Source: CAD feature listing. Evaluate the final solid. Frame: model axes, mm. Face numbers are marked on the shaded views. A direction names the side the tool comes from. Give positions to 0.01 mm unless a question says otherwise; leave off trailing zeros. Write each loop counter-clockwise with the first axis right and the second up, starting at its lowest first coordinate (ties: lowest second). Pieces come first, ordered by that corner, then holes.
```python
from build123d import *

# Parameters (mm, degrees)
SKETCH1_W                = 52
SKETCH1_H                = 24
SKETCH1_R                = 8.25
BOSS_EXTRUDE1_DEPTH      = 12
SKETCH2_R                = 1
CUT_EXTRUDE1_DEPTH       = 32.048349393
SKETCH3_R                = 1.75
CUT_EXTRUDE2_DEPTH       = 1
CUT_EXTRUDE3_DEPTH       = 5
FILLET3_R                = 0.5
CHAMFER1_SIZE            = 2.5
SKETCH5_W                = 19
SKETCH5_H                = 12
BOSS_EXTRUDE2_DEPTH      = 8
SKETCH6_W                = 7
SKETCH6_H                = 19
BOSS_EXTRUDE3_DEPTH      = 24
CHAMFER2_SIZE            = 3
CHAMFER2_OF_MIRROR1_SIZE = 3


with BuildPart() as part:
    # Sketch1 → Boss-Extrude1 (new body)
    with BuildSketch(Plane(origin=(0, 0, 0), x_dir=(1, 0, 0), z_dir=(0, 1, 0))):
        Rectangle(SKETCH1_W, SKETCH1_H)
        with Locations(Location((12.75, 0, 0), (0, 0, 270))):
            Circle(SKETCH1_R, mode=Mode.SUBTRACT)
        with Locations(Location((-12.75, 0, 0), (0, 0, 270))):
            Circle(SKETCH1_R, mode=Mode.SUBTRACT)
    extrude(amount=BOSS_EXTRUDE1_DEPTH)

    # Sketch2 → Cut-Extrude1 (cut, through all)
    with BuildSketch(Plane(origin=(0, 12, 0), x_dir=(1, 0, 0), z_dir=(0, 1, 0))):
        with Locations(Location((-21.35, 8.85, 0), (0, 0, 270))):
            Circle(SKETCH2_R)
        with Locations(Location((21.35, 8.85, 0), (0, 0, 270))):
            Circle(SKETCH2_R)
        with Locations(Location((21.35, -8.85, 0), (0, 0, 270))):
            Circle(SKETCH2_R)
        with Locations(Location((-21.35, -8.85, 0), (0, 0, 270))):
            Circle(SKETCH2_R)
    extrude(amount=-CUT_EXTRUDE1_DEPTH, mode=Mode.SUBTRACT)

    # Sketch3 → Cut-Extrude2 (cut)
    with BuildSketch(Plane(origin=(0, 12, 0), x_dir=(1, 0, 0), z_dir=(0, 1, 0))):
        with Locations(Location((-21.35, 8.85, 0), (0, 0, 270))):
            Circle(SKETCH3_R)
        with Locations(Location((21.35, 8.85, 0), (0, 0, 270))):
            Circle(SKETCH3_R)
        with Locations(Location((21.35, -8.85, 0), (0, 0, 270))):
            Circle(SKETCH3_R)
        with Locations(Location((-21.35, -8.85, 0), (0, 0, 270))):
            Circle(SKETCH3_R)
    extrude(amount=-CUT_EXTRUDE2_DEPTH, mode=Mode.SUBTRACT)

    # Sketch4 → Cut-Extrude3 (cut)
    with BuildSketch(Plane.XZ):
        Polygon((-6, -5), (-6, -12), (6, -12), (6, -5), (0, -5), align=None)
    extrude(amount=-CUT_EXTRUDE3_DEPTH, mode=Mode.SUBTRACT)

    # Fillet3
    fillet3_edges = [part.edges().sort_by_distance(p)[0] for p in [
        (-6, 2.5, -5),
        (6, 5, -8.5),
        (6, 2.5, -5),
        (-6, 5, -8.5),
        (0, 5, -5),
    ]]
    fillet(fillet3_edges, radius=FILLET3_R)

    # Chamfer1
    chamfer1_edges = [part.edges().sort_by_distance(p)[0] for p in [
        (26, 6, 12),
        (-26, 6, 12),
        (-26, 6, -12),
        (26, 6, -12),
    ]]
    chamfer(chamfer1_edges, length=CHAMFER1_SIZE)

    # Sketch5 → Boss-Extrude2 (add)
    with BuildSketch(Plane.ZY.offset(26)):
        with Locations((0, 6)):
            Rectangle(SKETCH5_W, SKETCH5_H)
    boss_extrude2 = extrude(amount=BOSS_EXTRUDE2_DEPTH)

    # Sketch6 → Boss-Extrude3 (add)
    with BuildSketch(Plane.XZ):
        with Locations((-30.5, 0)):
            Rectangle(SKETCH6_W, SKETCH6_H)
    boss_extrude3 = extrude(amount=BOSS_EXTRUDE3_DEPTH)

    # Chamfer2
    chamfer2_edges = [part.edges().sort_by_distance(p)[0] for p in [
        (-34, -6, 9.5),
        (-34, 12, 0),
        (-34, -6, -9.5),
    ]]
    chamfer(chamfer2_edges, length=CHAMFER2_SIZE)

    # Mirror1: Boss-Extrude2, Boss-Extrude3 across plane
    add(boss_extrude2.mirror(Plane(origin=(0, 0, 0), x_dir=(0, 0, 1), z_dir=(1, 0, 0))))
    add(boss_extrude3.mirror(Plane(origin=(0, 0, 0), x_dir=(0, 0, 1), z_dir=(1, 0, 0))))

    # Chamfer2 of Mirror1
    chamfer2_of_mirror1_edges = [part.edges().sort_by_distance(p)[0] for p in [
        (34, -6, 9.5),
        (34, 12, 0),
        (34, -6, -9.5),
    ]]
    chamfer(chamfer2_of_mirror1_edges, length=CHAMFER2_OF_MIRROR1_SIZE)


solid = part.part
```
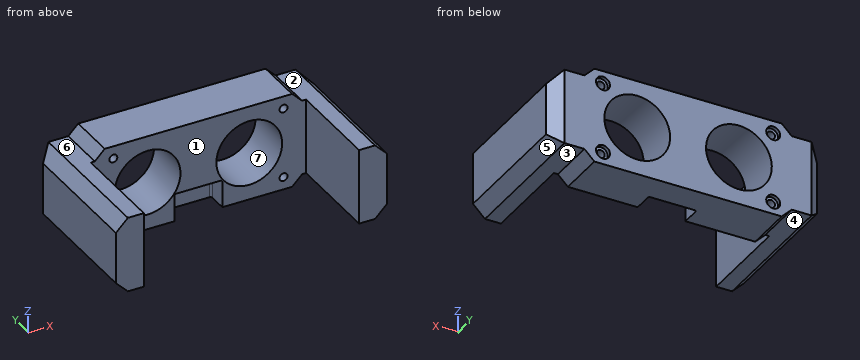
1. Pin query (flat end, axial travel): P1, Ø1.3, axis at y = 1.5, z = -8, coming from the +X side; P2, Ø2.5, axis at x = -21.35, z = -8.85, coming from the -Y side; P3, Ø2.5, axis at x = -21.35, z = 8.85, coming from the +Y side; P4, Ø1.8, axis at x = 22, z = -8, coming from the +Y side. Return the tip coordinate at first contact, or that it passes through.
2. Section query B-B (z = 0). Return loops of the section in (x, y), plus the area to 3 significant figures.
3. Pull-direction query (Z, two-part tool) for the marked faces 5, 6 and 7; classes: pulls with the +Z half, pulls with the -Z half, needs draft (parallel to the pull), parting line crosses it, or undercut.
4. Section query C-C (x = 12.75). Return loops of the section in (y, z), plus the area to 3 significant figures.
5. Section query D-D (x = 1.5). Return loops of the section in (y, z), plus the area to 3 significant figures.
6. Line query: probe 1 along X at (y, z) = (4.75, 0); probe 2 along X at (y, z) = (-14, -5.5); probe 3 along X at (y, z) = (5.75, -8.85). Output: solid intervals per line, ascending.
7. Access query for the marked faces 1, 2, 3 and 4. Directions: +Z, -Z, +X, -X, +Y, -Y. A direction counts if a zero-diameter tool reaches every point of the face in a straight line with its end or side. Return the directions, or none.
8. Section query A-A (y = -9). Return loops of the section in (x, z), plus the area to 3 significant figures.
The answers:
1. P1: stops at x = 33.15
1. P2: stops at y = 0
1. P3: stops at y = 11
1. P4: stops at y = 12
2. outline: (-34, -24) - (-27, -24) - (-27, 0) - (-21, 0) - (-21, 12) - (-31, 12) - (-34, 9) - close; (-4.5, 0) - (4.5, 0) - (4.5, 12) - (-4.5, 12) - close; (21, 0) - (27, 0) - (27, -24) - (34, -24) - (34, 9) - (31, 12) - (21, 12) - close
2. area: 747 mm2
3. face 5: pulls with the -Z half
3. face 6: pulls with the +Z half
3. face 7: undercut
4. outline: (0, -12) - (12, -12) - (12, -8.25) - (0, -8.25) - close; (0, 8.25) - (12, 8.25) - (12, 12) - (0, 12) - close
4. area: 90.0 mm2
5. outline: (0, -5) - (4.5, -5) arc R0.5 cw to (5, -5.5) - (5, -12) - (12, -12) - (12, 12) - (0, 12) - close
5. area: 253 mm2
6. probe 1: x = -34 to -21, -4.5 to 4.5, 21 to 34
6. probe 2: x = -34 to -27, 27 to 34
6. probe 3: x = -31.65 to -22.35, -20.35 to 20.35, 22.35 to 31.65
7. face 1: +Z, -Z, -Y
7. face 2: +Z, +X, +Y, -Y
7. face 3: -Z, +X, +Y, -Y
7. face 4: -Z, -X, +Y, -Y
8. outline: (-34, -6.5) - (-31, -9.5) - (-27, -9.5) - (-27, 9.5) - (-31, 9.5) - (-34, 6.5) - close; (27, -9.5) - (31, -9.5) - (34, -6.5) - (34, 6.5) - (31, 9.5) - (27, 9.5) - close
8. area: 248 mm2
